from build123d import *

# Parameters (mm, degrees)
SKETCH1_W           = 76.2
SKETCH1_H           = 152.4
BOSS_EXTRUDE1_DEPTH = 6.35
SKETCH3_W           = 76.2
SKETCH3_H           = 6.35
BOSS_EXTRUDE2_DEPTH = 101.6
SKETCH4_R           = 1.905
CUT_EXTRUDE1_DEPTH  = 191.605803952
SKETCH5_R           = 1.397
CUT_EXTRUDE2_DEPTH  = 182.94716953


with BuildPart() as part:
    # Sketch1 → Boss-Extrude1 (new body)
    with BuildSketch(Plane.XY):
        with Locations((0, 76.2)):
            Rectangle(SKETCH1_W, SKETCH1_H)
    extrude(amount=BOSS_EXTRUDE1_DEPTH)

    # Sketch3 → Boss-Extrude2 (add)
    with BuildSketch(Plane.XY):
        with Locations((0, 3.175)):
            Rectangle(SKETCH3_W, SKETCH3_H)
    extrude(amount=-BOSS_EXTRUDE2_DEPTH)

    # Sketch4 → Cut-Extrude1 (cut, through all)
    with BuildSketch(Plane.XY.offset(6.35)):
        with Locations((21.59, 76.2)):
            Circle(SKETCH4_R)
        with Locations((21.59, 12.7)):
            Circle(SKETCH4_R)
        with Locations((-21.59, 12.7)):
            Circle(SKETCH4_R)
        with Locations((-21.59, 76.2)):
            Circle(SKETCH4_R)
        with Locations((21.336, 140.208)):
            Circle(SKETCH4_R)
        with Locations((-21.59, 140.208)):
            Circle(SKETCH4_R)
    extrude(amount=-CUT_EXTRUDE1_DEPTH, mode=Mode.SUBTRACT)

    # Sketch5 → Cut-Extrude2 (cut, through all)
    with BuildSketch(Plane(origin=(0, 6.35, 0), x_dir=(1, 0, 0), z_dir=(0, 1, 0))):
        with BuildLine():
            ThreePointArc((-28.956, 92.456), (-27.968171827, 92.865171827), (-27.559, 93.853))
            Line((-27.559, 93.853), (-28.956, 93.853))
            Line((-28.956, 93.853), (-28.956, 92.456))
        make_face()
        with BuildLine():
            Line((-28.956, 93.853), (-27.559, 93.853))
            ThreePointArc((-27.559, 93.853), (-29.943828173, 94.840828173), (-28.956, 92.456))
            Line((-28.956, 92.456), (-28.956, 93.853))
        make_face()
        with BuildLine():
            ThreePointArc((30.353, 93.853), (28.956, 95.25), (27.559, 93.853))
            Line((27.559, 93.853), (28.956, 93.853))
            Line((28.956, 93.853), (28.956, 92.456))
            ThreePointArc((28.956, 92.456), (29.943828173, 92.865171827), (30.353, 93.853))
        make_face()
        with BuildLine():
            Line((28.956, 93.853), (27.559, 93.853))
            ThreePointArc((27.559, 93.853), (27.968171827, 92.865171827), (28.956, 92.456))
            Line((28.956, 92.456), (28.956, 93.853))
        make_face()
        with Locations(Location((-28.956, 7.747, 0), (0, 0, 90))):
            Circle(SKETCH5_R)
        with Locations(Location((28.956, 7.747, 0), (0, 0, 270))):
            Circle(SKETCH5_R)
    extrude(amount=-CUT_EXTRUDE2_DEPTH, mode=Mode.SUBTRACT)


solid = part.part
CAD build for the part. Positions are in the model's coordinates, mm. A direction names the side the tool comes from. Round coordinates to 2 decimals unless told otherwise and drop trailing zeros. Write each loop counter-clockwise with the first axis right and the second up, starting at its lowest first coordinate (ties: lowest second). Pieces come first, ordered by that corner, then holes. Notation, with made-up numbers: M 73,43.25 L 84,43.25 A36 ccw 84,77.25 Z; hole C -21.5,-26 d7. An arc over 180 degrees is marked long. Put each result on its own line as item: value. Start each with the question number.
1) Drill centre lines: probe 1 along Y at (x, z) = (21.59, 1.5) (3 decimals); probe 2 along Y at (x, z) = (-21, 2); probe 3 along Z at (x, y) = (18.5, 136.5). Where is each one in solid material? Low to high. Write a range as [from, to].
2) 3-axis set-ups, long thin cutter, end or side, ignore diameter. For faces 4 (the flat face through (38.1, 53, 1)), 5 (the flat face through (-1, 6.35, -50)): which of +Z, -Z, +X, -X, +Y, -Y reach the whole face in a straight line?
3) Saw through at A-A, the plane y = 12.7. Write the cut outline in (x, z) (3 decimals).
4) Pin check, flat tips, straight feed: pin 1 Ø3 at (x, z) = (-4.5, -29.5) entering from +Y; pin 2 Ø3 at (x, y) = (-21.5, 86.5) entering from -Z. Stop position of each tip, or through.
5) Saw through at B-B, the plane x = -21.59. Write the cut outline in (y, z) (3 decimals), and give its area (3 significant figures).
6) Saw through at C-C, the plane x = 16. Write the cut outline in (y, z).
7) Pull direction Y, two halves, no side cores. Call faces 1 (the flat face through (-1, 152.4, 3)), 2 (the flat face through (-1, 3, -101.6)), 3 (the cylindrical face through (-21.8, 142.1, 3.2)): pulls with the +Y half, pulls with the -Y half, needs draft (parallel to the pull), parting line crosses it, or undercut.
8) Saw through at D-D, the plane y = 114. Write the cut outline in (x, z).
Resolved:
1. probe 1: [0, 10.795], [14.605, 74.295], [78.105, 138.32], [142.096, 152.4]
1. probe 2: [0, 10.89], [14.51, 74.39], [78.01, 138.4], [142.02, 152.4]
1. probe 3: [0, 6.35]
2. face 4: +Z, -Z, +X, +Y, -Y
2. face 5: -Z, +X, -X, +Y
3. outline: M -38.1,0 L -23.495,0 L -23.495,6.35 L -38.1,6.35 Z; M -19.685,0 L 19.685,0 L 19.685,6.35 L -19.685,6.35 Z; M 23.495,0 L 38.1,0 L 38.1,6.35 L 23.495,6.35 Z
4. pin 1: y = 6.35
4. pin 2: z = 0
5. outline: M 0,-101.6 L 6.35,-101.6 L 6.35,0 L 10.795,0 L 10.795,6.35 L 0,6.35 Z; M 14.605,0 L 74.295,0 L 74.295,6.35 L 14.605,6.35 Z; M 78.105,0 L 138.303,0 L 138.303,6.35 L 78.105,6.35 Z; M 142.113,0 L 152.4,0 L 152.4,6.35 L 142.113,6.35 Z
5. area: 1,540 mm²
6. outline: M 0,-101.6 L 6.35,-101.6 L 6.35,0 L 152.4,0 L 152.4,6.35 L 0,6.35 Z
7. face 1: pulls with the +Y half
7. face 2: needs draft
7. face 3: undercut
8. outline: M -38.1,0 L 38.1,0 L 38.1,6.35 L -38.1,6.35 Z
